from build123d import *

# Parameters (mm, degrees)
SKETCH1_W           = 90
SKETCH1_H           = 95
BOSS_EXTRUDE3_DEPTH = 15
SKETCH5_W           = 15
SKETCH5_H           = 8.4
CUT_EXTRUDE3_DEPTH  = 40
SKETCH7_W           = 95
SKETCH7_H           = 15
BOSS_EXTRUDE4_DEPTH = 5
CUT_EXTRUDE4_DEPTH  = 100
FILLET6_R           = 17


with BuildPart() as part:
    # Sketch1 → Boss-Extrude3 (new body)
    with BuildSketch(Plane(origin=(0, 0, 0), x_dir=(1, 0, 0), z_dir=(0, 1, 0))):
        Rectangle(SKETCH1_W, SKETCH1_H)
    extrude(amount=BOSS_EXTRUDE3_DEPTH)

    # Sketch5 → Cut-Extrude3 (cut)
    with BuildSketch(Plane(origin=(45, 0, 0), x_dir=(0, 0, -1), z_dir=(1, 0, 0))):
        with Locations((0.9, 6.2)):
            Rectangle(SKETCH5_W, SKETCH5_H)
    extrude(amount=-CUT_EXTRUDE3_DEPTH, mode=Mode.SUBTRACT)

    # Sketch7 → Boss-Extrude4 (add)
    with BuildSketch(Plane(origin=(45, 0, 0), x_dir=(0, 0, -1), z_dir=(1, 0, 0))):
        with Locations((0, 7.5)):
            Rectangle(SKETCH7_W, SKETCH7_H)
    extrude(amount=BOSS_EXTRUDE4_DEPTH)

    # Sketch8 → Cut-Extrude4 (cut)
    with BuildSketch(Plane.XY.offset(47.5)):
        Polygon((42.5, 2.5), (50, 0), (50, 15), (35, 15), align=None)
    extrude(amount=-CUT_EXTRUDE4_DEPTH, mode=Mode.SUBTRACT)

    # Fillet6
    # the kernel refuses this fillet: 17 mm, written as the material it adds along each edge
    with BuildSketch(Plane(origin=(42.5, 2.5, 7.321773239), x_dir=(0.9486832980505139, -0.316227766016838, 0), z_dir=(0, 0, -1))) as fillet6_piece_1_section:
        with BuildLine():
            CenterArc((FILLET6_R * 0.369924076215, -FILLET6_R), FILLET6_R, 90, 40.601294645)
            Line((-FILLET6_R * 0.28086729724, -FILLET6_R * 0.240743397635), (0, 0))
            Line((0, 0), (FILLET6_R * 0.369924076215, 0))
        make_face()
    fillet6_piece_1 = extrude(amount=54.821773239, mode=Mode.PRIVATE)
    fillet6_piece_1 = split(fillet6_piece_1, bisect_by=Plane(origin=(45.830299546, 2, 6.96088662), z_dir=(0, -1, 0)), keep=Keep.TOP, mode=Mode.PRIVATE)
    fillet6_piece_1 = split(fillet6_piece_1, bisect_by=Plane(origin=(45.830299546, 1.289116615, 6.6), z_dir=(0, 0, 1)), keep=Keep.TOP, mode=Mode.PRIVATE)
    add(fillet6_piece_1)
    with BuildSketch(Plane(origin=(42.5, 2.5, 7.321773239), x_dir=(0.9486832980505139, -0.316227766016838, 0), z_dir=(0, 0, -1))) as fillet6_piece_2_section:
        with BuildLine():
            CenterArc((FILLET6_R * 0.369924076215, -FILLET6_R), FILLET6_R, 90, 40.601294645)
            Line((-FILLET6_R * 0.28086729724, -FILLET6_R * 0.240743397635), (0, 0))
            Line((0, 0), (FILLET6_R * 0.369924076215, 0))
        make_face()
    fillet6_piece_2 = extrude(amount=54.821773239, mode=Mode.PRIVATE)
    fillet6_piece_2 = split(fillet6_piece_2, bisect_by=Plane(origin=(42.01228151, 2, 6.96088662), z_dir=(0, 1, 0)), keep=Keep.TOP, mode=Mode.PRIVATE)
    fillet6_piece_2 = split(fillet6_piece_2, bisect_by=Plane(origin=(42.01228151, 3.937960854, 6.6), z_dir=(0, 0, 1)), keep=Keep.TOP, mode=Mode.PRIVATE)
    add(fillet6_piece_2)
    with BuildSketch(Plane(origin=(42.5, 2.5, 7.321773239), x_dir=(0.9486832980505139, -0.316227766016838, 0), z_dir=(0, 0, -1))) as fillet6_piece_3_section:
        with BuildLine():
            CenterArc((FILLET6_R * 0.369924076215, -FILLET6_R), FILLET6_R, 90, 40.601294645)
            Line((-FILLET6_R * 0.28086729724, -FILLET6_R * 0.240743397635), (0, 0))
            Line((0, 0), (FILLET6_R * 0.369924076215, 0))
        make_face()
    fillet6_piece_3 = extrude(amount=54.821773239, mode=Mode.PRIVATE)
    fillet6_piece_3 = split(fillet6_piece_3, bisect_by=Plane(origin=(45.830299546, 1.289116615, -8.4), z_dir=(0, 0, 1)), keep=Keep.TOP, mode=Mode.PRIVATE)
    fillet6_piece_3 = split(fillet6_piece_3, bisect_by=Plane(origin=(45.830299546, 2, -0.9), z_dir=(0, -1, 0)), keep=Keep.TOP, mode=Mode.PRIVATE)
    fillet6_piece_3 = split(fillet6_piece_3, bisect_by=Plane(origin=(45.830299546, 1.289116615, 6.6), z_dir=(0, 0, -1)), keep=Keep.TOP, mode=Mode.PRIVATE)
    add(fillet6_piece_3)
    with BuildSketch(Plane(origin=(42.5, 2.5, -8.4), x_dir=(0.9486832980505139, -0.316227766016838, 0), z_dir=(0, 0, -1))) as fillet6_piece_4_section:
        with BuildLine():
            CenterArc((FILLET6_R * 0.369924076215, -FILLET6_R), FILLET6_R, 90, 40.601294645)
            Line((-FILLET6_R * 0.28086729724, -FILLET6_R * 0.240743397635), (0, 0))
            Line((0, 0), (FILLET6_R * 0.369924076215, 0))
        make_face()
    fillet6_piece_4 = extrude(amount=39.1, mode=Mode.PRIVATE)
    fillet6_piece_4 = split(fillet6_piece_4, bisect_by=Plane(origin=(45.830299546, 2, -27.95), z_dir=(0, -1, 0)), keep=Keep.TOP, mode=Mode.PRIVATE)
    add(fillet6_piece_4)
    with BuildSketch(Plane(origin=(42.5, 2.5, -8.4), x_dir=(0.9486832980505139, -0.316227766016838, 0), z_dir=(0, 0, -1))) as fillet6_piece_5_section:
        with BuildLine():
            CenterArc((FILLET6_R * 0.369924076215, -FILLET6_R), FILLET6_R, 90, 40.601294645)
            Line((-FILLET6_R * 0.28086729724, -FILLET6_R * 0.240743397635), (0, 0))
            Line((0, 0), (FILLET6_R * 0.369924076215, 0))
        make_face()
    fillet6_piece_5 = extrude(amount=39.1, mode=Mode.PRIVATE)
    fillet6_piece_5 = split(fillet6_piece_5, bisect_by=Plane(origin=(42.01228151, 2, -27.95), z_dir=(0, 1, 0)), keep=Keep.TOP, mode=Mode.PRIVATE)
    add(fillet6_piece_5)
    with BuildSketch(Plane(origin=(42.5, 2.5, 47.5), x_dir=(0.9486832980505139, -0.316227766016838, 0), z_dir=(0, 0, -1))) as fillet6_piece_6_section:
        with BuildLine():
            CenterArc((FILLET6_R * 0.369924076215, -FILLET6_R), FILLET6_R, 90, 40.601294645)
            Line((-FILLET6_R * 0.28086729724, -FILLET6_R * 0.240743397635), (0, 0))
            Line((0, 0), (FILLET6_R * 0.369924076215, 0))
        make_face()
    fillet6_piece_6 = extrude(amount=40.9, mode=Mode.PRIVATE)
    fillet6_piece_6 = split(fillet6_piece_6, bisect_by=Plane(origin=(45.830299546, 2, 27.05), z_dir=(0, -1, 0)), keep=Keep.TOP, mode=Mode.PRIVATE)
    add(fillet6_piece_6)
    with BuildSketch(Plane(origin=(42.5, 2.5, 47.5), x_dir=(0.9486832980505139, -0.316227766016838, 0), z_dir=(0, 0, -1))) as fillet6_piece_7_section:
        with BuildLine():
            CenterArc((FILLET6_R * 0.369924076215, -FILLET6_R), FILLET6_R, 90, 40.601294645)
            Line((-FILLET6_R * 0.28086729724, -FILLET6_R * 0.240743397635), (0, 0))
            Line((0, 0), (FILLET6_R * 0.369924076215, 0))
        make_face()
    fillet6_piece_7 = extrude(amount=40.9, mode=Mode.PRIVATE)
    fillet6_piece_7 = split(fillet6_piece_7, bisect_by=Plane(origin=(42.01228151, 2, 27.05), z_dir=(0, 1, 0)), keep=Keep.TOP, mode=Mode.PRIVATE)
    add(fillet6_piece_7)
    with BuildSketch(Plane(origin=(42.5, 2.5, 47.5), x_dir=(0.9486832980505139, -0.316227766016838, 0), z_dir=(0, 0, -1))) as fillet6_piece_8_section:
        with BuildLine():
            CenterArc((FILLET6_R * 0.369924076215, -FILLET6_R), FILLET6_R, 90, 40.601294645)
            Line((-FILLET6_R * 0.28086729724, -FILLET6_R * 0.240743397635), (0, 0))
            Line((0, 0), (FILLET6_R * 0.369924076215, 0))
        make_face()
    fillet6_piece_8 = extrude(amount=56.621773239, mode=Mode.PRIVATE)
    fillet6_piece_8 = split(fillet6_piece_8, bisect_by=Plane(origin=(45.830299546, 1.289116615, -8.4), z_dir=(0, 0, 1)), keep=Keep.TOP, mode=Mode.PRIVATE)
    fillet6_piece_8 = split(fillet6_piece_8, bisect_by=Plane(origin=(45.830299546, 2, -0.9), z_dir=(0, -1, 0)), keep=Keep.TOP, mode=Mode.PRIVATE)
    fillet6_piece_8 = split(fillet6_piece_8, bisect_by=Plane(origin=(45.830299546, 1.289116615, 6.6), z_dir=(0, 0, -1)), keep=Keep.TOP, mode=Mode.PRIVATE)
    add(fillet6_piece_8)
    with BuildSketch(Plane(origin=(42.5, 2.5, 47.5), x_dir=(0.9486832980505139, -0.316227766016838, 0), z_dir=(0, 0, -1))) as fillet6_piece_9_section:
        with BuildLine():
            CenterArc((FILLET6_R * 0.369924076215, -FILLET6_R), FILLET6_R, 90, 40.601294645)
            Line((-FILLET6_R * 0.28086729724, -FILLET6_R * 0.240743397635), (0, 0))
            Line((0, 0), (FILLET6_R * 0.369924076215, 0))
        make_face()
    fillet6_piece_9 = extrude(amount=56.621773239, mode=Mode.PRIVATE)
    fillet6_piece_9 = split(fillet6_piece_9, bisect_by=Plane(origin=(45.830299546, 1.289116615, -8.4), z_dir=(0, 0, -1)), keep=Keep.TOP, mode=Mode.PRIVATE)
    fillet6_piece_9 = split(fillet6_piece_9, bisect_by=Plane(origin=(45.830299546, 2, -8.76088662), z_dir=(0, -1, 0)), keep=Keep.TOP, mode=Mode.PRIVATE)
    add(fillet6_piece_9)
    with BuildSketch(Plane(origin=(42.5, 2.5, 47.5), x_dir=(0.9486832980505139, -0.316227766016838, 0), z_dir=(0, 0, -1))) as fillet6_piece_10_section:
        with BuildLine():
            CenterArc((FILLET6_R * 0.369924076215, -FILLET6_R), FILLET6_R, 90, 40.601294645)
            Line((-FILLET6_R * 0.28086729724, -FILLET6_R * 0.240743397635), (0, 0))
            Line((0, 0), (FILLET6_R * 0.369924076215, 0))
        make_face()
    fillet6_piece_10 = extrude(amount=56.621773239, mode=Mode.PRIVATE)
    fillet6_piece_10 = split(fillet6_piece_10, bisect_by=Plane(origin=(42.01228151, 3.937960854, -8.4), z_dir=(0, 0, -1)), keep=Keep.TOP, mode=Mode.PRIVATE)
    fillet6_piece_10 = split(fillet6_piece_10, bisect_by=Plane(origin=(42.01228151, 2, -8.76088662), z_dir=(0, 1, 0)), keep=Keep.TOP, mode=Mode.PRIVATE)
    add(fillet6_piece_10)


solid = part.part
Here's how the part is built. I have some questions about the finished solid (model axes, mm). A direction names the side the tool comes from. Coordinates: 2 decimals unless noted, no trailing zeros. Order: outer loops, then holes, each group sorted by start corner. A loop starts at its lowest first (then second) coordinate and runs counter-clockwise, first axis right, second up.
Item 1: For P1, Ø5, axis at y = 10, z = 29.5, coming from the +X side; P2, Ø4, axis at y = 7, z = 0, coming from the +X side, each with a flat end and sliding along its axis, tell me the tip position at first contact or that it passes through.
Result sheet:
P1: stops at x = 39.51
P2: stops at x = 5
Item 2: If we section it at B-B on z = 2.5: List the corners of the cut face in (x, y) for me.
Result sheet:
outline: (-45, 0) - (50, 0) - (48.47, 0.51) arc R17 cw to (45.2, 2) - (5, 2) - (5, 10.4) - (37.76, 10.4) - (35, 15) - (-45, 15) - close
Item 3: If we section it at A-A on x = 18.5: List the corners of the cut face in (y, z) for me.
Result sheet:
outline: (0, -47.5) - (15, -47.5) - (15, 47.5) - (0, 47.5) - close; hole (2, -8.4) - (10.4, -8.4) - (10.4, 6.6) - (2, 6.6) - close
Item 4: I need wall thicknesses on line 1 (Z direction, x = 7, y = 3.75); line 2 (X direction, y = 6, z = -5); line 3 (X direction, y = 6.25, z = 38). Which ranges of each line are inside material? Lowest first, please.
Result sheet:
line 1: z = -47.5 to -8.4, 6.6 to 47.5
line 2: x = -45 to 5
line 3: x = -45 to 40.39
Item 5: If we section it at C-C on y = 12: List the corners of the cut face in (x, z) for me.
Result sheet:
outline: (-45, -47.5) - (36.8, -47.5) - (36.8, 47.5) - (-45, 47.5) - close
Item 6: For faces 4 (the face through (-6, 15, 1)), 5 (the face through (22, 10.4, -1)), which set-ups out of +Z, -Z, +X, -X, +Y, -Y let a thin tool reach every point of the face, with its end or its side?
Result sheet:
face 4: +Z, -Z, +X, -X, +Y
face 5: +X
Item 7: If we section it at D-D on y = 4.5: List the corners of the cut face in (x, z) for me, plus the area to 3 significant figures.
Result sheet:
outline: (-45, -47.5) - (41.94, -47.5) - (41.94, -8.4) - (5, -8.4) - (5, 6.6) - (41.94, 6.6) - (41.94, 47.5) - (-45, 47.5) - close
area: 7,710 mm2
Item 8: If we mould it in two halves opening along Y, with no side actions, what happens to faces 1 (the face through (25, 5, -8.4)), 2 (the face through (2, 0, 1)), 3 (the face through (0, 9, 47.5))? For each: +Y half, -Y half, draft (parallel to the pull), parting line (faces both ways), or undercut.
Result sheet:
face 1: undercut
face 2: -Y half
face 3: draft
